```python
from build123d import *

# Parameters (mm, degrees)
F2_DEPTH = 5


with BuildPart() as f2:
    # F1 (on Front) → F2 (new body)
    with BuildSketch(Plane.XZ):
        Polygon((-30, 0), (0, 0), (0, 10), (5, 10), (5, 20), (0, 20), (0, 28.4), (-2.5, 28.4), (-2.5, 27.25), (-5, 27.25), (-5, 30), (-5, 32.75), (-2.5, 32.75), (-2.5, 31.6), (0, 31.6), (0, 40), (5, 40), (5, 50), (0, 50), (0, 60), (-12.5, 60), (-12.5, 65), (-22.5, 65), (-22.5, 60), (-30.9, 60), (-30.9, 57.5), (-29.75, 57.5), (-29.75, 55), (-32.5, 55), (-35.25, 55), (-35.25, 57.5), (-34.1, 57.5), (-34.1, 60), (-42.5, 60), (-42.5, 65), (-52.5, 65), (-52.5, 60), (-57.5, 60), (-57.5, 55), align=None)
    extrude(amount=F2_DEPTH)


solid = f2.part
```
Check sheet for the modelled part. Datum: model origin and axes. Units: mm. A direction names the side the tool comes from. Round coordinates to 2 decimals unless told otherwise and drop trailing zeros. Order: outer loops, then holes, each group sorted by start corner. A loop starts at its lowest first (then second) coordinate and runs counter-clockwise, first axis right, second up.
1) Mould release check, pull along Z, two halves, no side actions. Record for faces 5 (the flat face through (5, -2, 15)), 6 (the flat face through (3, -2, 50)), 7 (the flat face through (-4, -2, 27.25)): +Z half, -Z half, draft (parallel to the pull), parting line (faces both ways), or undercut.
2) Section check B-B (x = -51). Record the boundary of the cut face in (y, z).
3) Section check A-A (z = 45). Record the boundary of the cut face in (x, y).
4) Tool access check on faces 1 (the flat face through (-30.9, -2, 59)), 2 (the flat face through (-4, -2, 32.75)), 3 (the flat face through (0, -2, 36)), 4 (the flat face through (0, -2, 55)). Record the directions out of +Z, -Z, +X, -X, +Y, -Y that give a thin tool (end or side, any length) a straight path to the whole face; none if there is none.
5) Go/stop test with flat-tipped pins: pin 1 Ø1.5 at (y, z) = (-3, 63) entering from +X; pin 2 Ø1.5 at (x, y) = (3.5, -2) entering from -Z; pin 3 Ø2 at (y, z) = (-1.5, 55.5) entering from +X. Record where each tip stops, or that it passes through.
6) Scan lines: line 1 (Z direction, x = -1, y = -0.45); line 2 (Z direction, x = -4.5, y = -2.2); line 3 (X direction, y = -2.4, z = 58.5). Record each from-to range of solid material in increasing order.
Result:
1. face 5: draft
1. face 6: +Z half
1. face 7: undercut
2. outline: (-5, 42) - (0, 42) - (0, 65) - (-5, 65) - close
3. outline: (-52.5, -5) - (5, -5) - (5, 0) - (-52.5, 0) - close
4. face 1: +Z, +Y, -Y
4. face 2: +Y, -Y
4. face 3: +X, +Y, -Y
4. face 4: +Z, +X, +Y, -Y
5. pin 1: stops at x = -12.5
5. pin 2: stops at z = 10
5. pin 3: stops at x = 0
6. line 1: z = 0 to 28.4, 31.6 to 60
6. line 2: z = 0 to 27.25, 32.75 to 60
6. line 3: x = -57.5 to -34.1, -30.9 to 0
